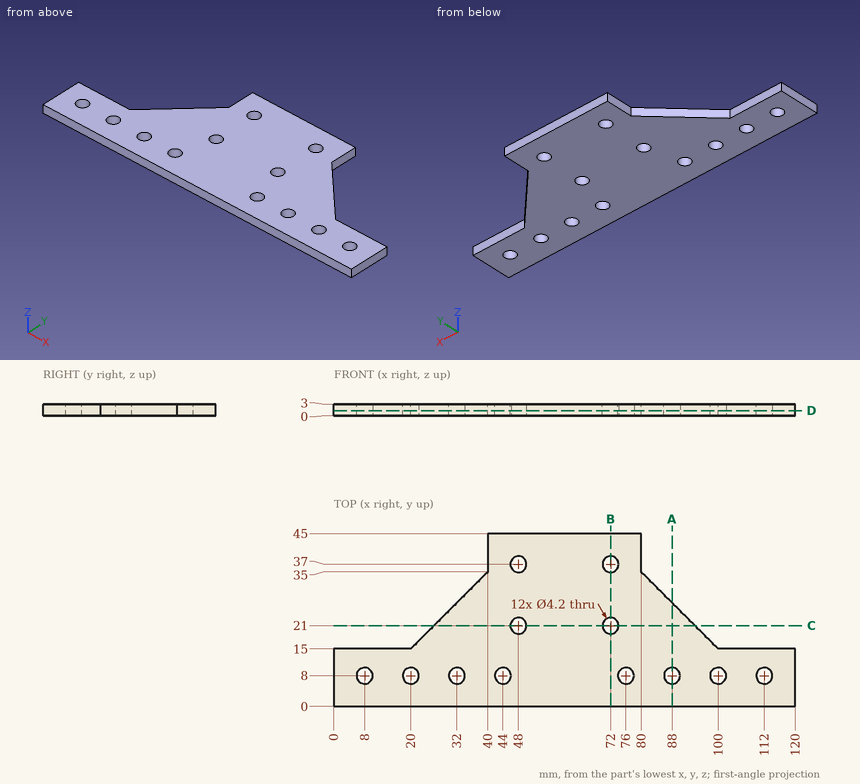
The figure shows three views and two pictorial views of one solid part (mm, origin at its lowest corner). Answer the questions. Coordinates: 2 decimals unless noted, no trailing zeros. Write each loop counter-clockwise with the first axis right and the second up, starting at its lowest first coordinate (ties: lowest second). Pieces come first, ordered by that corner, then holes.
1. The part is cut by section B-B, the plane x = 72. Write down the section's boundary in (y, z).
Results list:
outline: (0, 0) - (18.9, 0) - (18.9, 3) - (0, 3) - close; (23.1, 0) - (34.9, 0) - (34.9, 3) - (23.1, 3) - close; (39.1, 0) - (45, 0) - (45, 3) - (39.1, 3) - close
2. The part is cut by section D-D, the plane z = 1.25. State how many separate pieces and enclosed holes the cut face has, and give its area (3 significant figures).
Results list:
separate pieces: 1
enclosed holes: 12
area: 3,230 mm2
3. Consider line 1 along Y through (x, z) = (100, 1.55); line 2 along Y through (x, z) = (99, 2.3); line 3 along X through (y, z) = (42, 2.2). Determine where each line is inside the solid, lowest interval first.
Results list:
line 1: y = 0 to 5.9, 10.1 to 15
line 2: y = 0 to 6.15, 9.85 to 16
line 3: x = 40 to 80
4. The part is cut by section C-C, the plane y = 21. Write down the section's boundary in (x, z), and give its area (3 significant figures).
Results list:
outline: (26, 0) - (45.9, 0) - (45.9, 3) - (26, 3) - close; (50.1, 0) - (69.9, 0) - (69.9, 3) - (50.1, 3) - close; (74.1, 0) - (94, 0) - (94, 3) - (74.1, 3) - close
area: 179 mm2
5. Flat-ended cylindrical pins translate along their axes: pin 1 (0.9 mm diameter, centred on x = 15, z = 2, fed in from +Y); pin 2 (1.5 mm diameter, centred on y = 41.5, z = 1, fed in from +X). Find the tip coordinate at first contact, or state that the pin passes through.
Results list:
pin 1: stops at y = 15
pin 2: stops at x = 80
6. The part is cut by section A-A, the plane x = 88. Write down the section's boundary in (y, z), and give its area (3 significant figures).
Results list:
outline: (0, 0) - (5.9, 0) - (5.9, 3) - (0, 3) - close; (10.1, 0) - (27, 0) - (27, 3) - (10.1, 3) - close
area: 68.4 mm2
